```python
from build123d import *

# Parameters (mm, degrees)
F1_DEPTH = 25
F3_DEPTH = 10
F4_SIZE  = 3
F6_DEPTH = 11


with BuildPart() as f1:
    # F0 (on Top) → F1 (new body)
    with BuildSketch(Plane.XY):
        Polygon((-25, 14.4337567297), (-25, -14.4337567297), (0, -28.8675134595), (25, -14.4337567297), (25, 14.4337567297), (0, 28.8675134595), align=None)
    extrude(amount=F1_DEPTH)

    # F2 (on face) → F3 (join)
    with BuildSketch(Plane.XY.offset(25)):
        with BuildLine():
            ThreePointArc((-12, 0), (0, -12), (12, 0))
            Line((12, 0), (-12, 0))
        make_face()
    extrude(amount=F3_DEPTH)

    # F4
    f4_edges = [f1.edges().sort_by_distance(p)[0] for p in [
        (0, 0, 35),
        (0, -12, 35),
    ]]
    chamfer(f4_edges, length=F4_SIZE)

    # F5 (on face) + F2 (on face) → F6 (cut)
    with BuildSketch(Plane.XY.offset(25)):
        with BuildLine():
            Line((12, 0), (12.5, 0))
            ThreePointArc((12.5, 0), (0, 12.5), (-12.5, 0))
            Line((-12.5, 0), (-12, 0))
            ThreePointArc((-12, 0), (0, 12), (12, 0))
        make_face()
    with BuildSketch(Plane.XY.offset(25)):
        with BuildLine():
            Line((-12, 0), (12, 0))
            ThreePointArc((12, 0), (0, 12), (-12, 0))
        make_face()
    extrude(amount=-F6_DEPTH, mode=Mode.SUBTRACT)


solid = f1.part
```
The listing builds one solid part. Answer for the finished solid, in the listing's coordinates (mm). A direction names the side the tool comes from. Round coordinates to 2 decimals unless told otherwise and drop trailing zeros. Loops run counter-clockwise (first coordinate to the right, second up) from the corner with the lowest first, then second, coordinate; pieces in that order, holes last.
1) A cutting plane is placed at D-D on x = -20. Determine the outline of the cut face in (y, z).
Outcome:
outline: (-17.32, 0) - (17.32, 0) - (17.32, 25) - (-17.32, 25) - close
2) A cutting plane is placed at B-B on y = 4.5. Determine the outline of the cut face in (x, z), plus the area to 3 significant figures.
Outcome:
outline: (-25, 0) - (25, 0) - (25, 25) - (11.66, 25) - (11.66, 14) - (-11.66, 14) - (-11.66, 25) - (-25, 25) - close
area: 993 mm2
3) Given P1, Ø14, axis at x = 4.5, y = 8.5, coming from the +Z side; P2, Ø1, axis at x = -13, z = 25, coming from the -Y side; P3, Ø1, axis at x = 6, z = 23, coming from the +Y side, each flat-ended and moving along its own axis, determine where each tip first touches the part or whether it passes through.
Outcome:
P1: stops at z = 25
P2: stops at y = -21.65
P3: stops at y = 25.69
4) For faces 1 (the face through (0.275, 12.497, 19.577)), 2 (the face through (25, 0, 12)), 3 (the face through (0, -12, 28)), determine the directions among +Z, -Z, +X, -X, +Y, -Y from which every point of the face is accessible in a straight line to the end or side of a thin tool.
Outcome:
face 1: +Z
face 2: +Z, -Z, +X, +Y, -Y
face 3: +Z, -Y
5) Consider line 1 (Z direction, x = 17, y = -19); line 2 (Y direction, x = 1, z = 20.5); line 3 (Z direction, x = 2, y = 6). Determine where each line is inside the solid, lowest interval first.
Outcome:
line 1: z = 0 to 25
line 2: y = -28.29 to 0, 12.46 to 28.29
line 3: z = 0 to 14
6) A cutting plane is placed at A-A on z = 16.5. Determine the outline of the cut face in (x, y), plus the area to 3 significant figures.
Outcome:
outline: (-25, -14.43) - (0, -28.87) - (25, -14.43) - (25, 14.43) - (0, 28.87) - (-25, 14.43) - close; hole (-12.5, 0) - (12.5, 0) arc R12.5 ccw to start
area: 1,920 mm2
7) A cutting plane is placed at C-C on z = 29. Determine the outline of the cut face in (x, y).
Outcome:
outline: (-12, 0) arc R12 ccw to (12, 0) - close
8) For a pull along Y with two mould halves and no side action, classify faces 4 (the face through (12.325, -21.752, 12.325)), 5 (the face through (0, -2, 34)), 6 (the face through (0, 5, 14)) as released by +Y, released by -Y, zero draft, split by the parting line, or undercut.
Outcome:
face 4: released by -Y
face 5: released by +Y
face 6: undercut
